For this review, take the finished solid that the model builds, in its own axes (mm). Face numbers are marked on the shaded views. A direction names the side the tool comes from. Coordinates: 2 decimals unless noted, no trailing zeros. Loops run counter-clockwise (first coordinate to the right, second up) from the corner with the lowest first, then second, coordinate; pieces in that order, holes last. Notation, with made-up numbers: (30.25, 15) - (63.25, 15) arc R37 cw to (63.25, 51) - close; hole circle Ø3 at (38.5, 46). An arc over 180 degrees is marked (long way). One line per item, written item: value. Start each with the question number.
1. The part is to be moulded in two halves that separate along Z. For the marked faces 3, 4 and 5, say which applies: released by +Z, released by -Z, zero draft, split by the parting line, or undercut.
2. Take a section at D-D, the plane x = 4.25. State the section outline as (y, z) points, and give its area (3 significant figures).
3. To check wall thickness, follow line 1 (X direction, y = 0.7, z = 5); line 2 (Z direction, x = -6.5, y = 1.35); line 3 (Z direction, x = -5, y = 2.6). State the ranges of each line that lie inside material, in increasing order. Write a range as from..to.
4. Take a section at B-B, the plane z = 5. Count the separate pieces of the cut face and the enclosed holes in it, and give its area (3 significant figures).
5. Take a section at C-C, the plane x = -1.25. State the section outline as (y, z) points, and give its area (3 significant figures).
6. Take a section at A-A, the plane y = 0.75. State the section outline as (x, z) points, and give its area (3 significant figures).
7. For the marked faces 1 and 2, list the 3-axis set-ups (+Z, -Z, +X, -X, +Y, -Y) from which the entire face can be reached by the end or side of a thin tool; tool diameter is ignored.
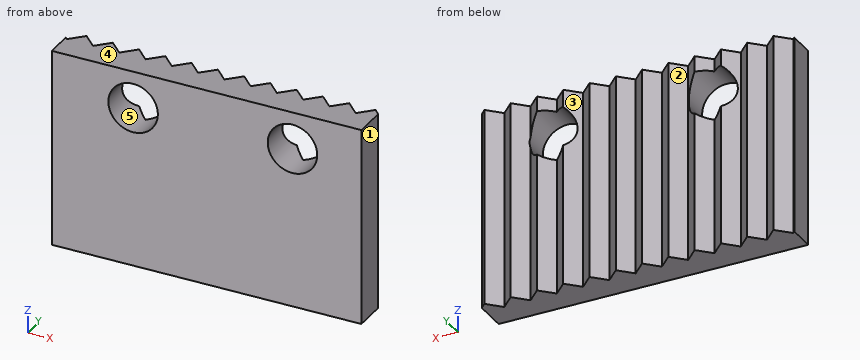
Autodesk Inventor part; units mm, degrees
ref_plane "YZ Plane" through (0, 0, 0) normal (1, 0, 0) x (0, 1, 0)
ref_plane "XZ Plane" through (0, 0, 0) normal (0, 1, 0) x (-1, 0, 0)
ref_plane "XY Plane" through (0, 0, 0) normal (0, 0, 1) x (1, 0, 0)
sketch "Sketch1" plane through (0, 0, 0) normal (0, 1, 0) x (-1, 0, 0)
  line L0 (24, 8) -> (-24, 8)
  line L1 (-24, 8) -> (-24, -8)
  line L2 (-24, -8) -> (24, -8)
  line L3 (24, -8) -> (24, 8)
  point P0 (0, 0)
  dimension "d0" = 48
  dimension "d1" = 16
extrude "Extrusion1" add sketch "Sketch1" along normal blind 2
sketch "Sketch2" plane through (-24, 0, 8) normal (0, 0, 1) x (1, 0, 0)
  line L0 (0, 2) -> (1.5, 2) construction
  line L1 (0, 3.0607) -> (1.0607, 2)
  line L2 (0, 2) -> (48, 2)
  line L3 (0, 3.0607) -> (0, 2)
  line L4 (1.0607, 2) -> (2.1213, 3.0607)
  line L5 (1.0607, 2) -> (2.5607, 2) construction
  line L6 (2.1213, 3.0607) -> (3.182, 2)
  line L7 (3.182, 2) -> (4.2426, 3.0607)
  line L8 (4.2426, 3.0607) -> (5.3033, 2)
  line L9 (5.3033, 2) -> (6.364, 3.0607)
  line L10 (6.364, 3.0607) -> (7.4246, 2)
  line L11 (7.4246, 2) -> (8.4853, 3.0607)
  line L12 (7.4246, 2) -> (8.9246, 2) construction
  line L13 (8.4853, 3.0607) -> (9.5459, 2)
  line L14 (9.5459, 2) -> (10.6066, 3.0607)
  line L15 (10.6066, 3.0607) -> (11.6673, 2)
  line L16 (11.6673, 2) -> (12.7279, 3.0607)
  line L17 (12.7279, 3.0607) -> (13.7886, 2)
  line L18 (13.7886, 2) -> (14.8492, 3.0607)
  line L19 (14.8492, 3.0607) -> (15.9099, 2)
  line L20 (15.9099, 2) -> (16.9706, 3.0607)
  line L21 (16.9706, 3.0607) -> (18.0312, 2)
  line L22 (18.0312, 2) -> (19.0919, 3.0607)
  line L23 (19.0919, 3.0607) -> (20.1525, 2)
  line L24 (20.1525, 2) -> (21.2132, 3.0607)
  line L25 (21.2132, 3.0607) -> (22.2739, 2)
  line L26 (22.2739, 2) -> (23.3345, 3.0607)
  line L27 (23.3345, 3.0607) -> (24.3952, 2)
  line L28 (24.3952, 2) -> (25.4558, 3.0607)
  line L29 (25.4558, 3.0607) -> (26.5165, 2)
  line L30 (26.5165, 2) -> (27.5772, 3.0607)
  line L31 (27.5772, 3.0607) -> (28.6378, 2)
  line L32 (27.5772, 3.0607) -> (29.0772, 3.0607) construction
  line L33 (28.6378, 2) -> (29.6985, 3.0607)
  line L34 (29.6985, 3.0607) -> (30.7591, 2)
  line L35 (30.7591, 2) -> (31.8198, 3.0607)
  line L36 (31.8198, 3.0607) -> (32.8805, 2)
  line L37 (32.8805, 2) -> (33.9411, 3.0607)
  line L38 (33.9411, 3.0607) -> (35.0018, 2)
  line L39 (35.0018, 2) -> (36.0624, 3.0607)
  line L40 (36.0624, 3.0607) -> (37.1231, 2)
  line L41 (37.1231, 2) -> (38.1838, 3.0607)
  line L42 (38.1838, 3.0607) -> (39.2444, 2)
  line L43 (39.2444, 2) -> (40.3051, 3.0607)
  line L44 (40.3051, 3.0607) -> (41.3657, 2)
  line L45 (41.3657, 2) -> (42.4264, 3.0607)
  line L46 (42.4264, 3.0607) -> (43.4871, 2)
  line L47 (43.4871, 2) -> (44.5477, 3.0607)
  line L48 (44.5477, 3.0607) -> (45.6084, 2)
  line L49 (45.6084, 2) -> (46.669, 3.0607)
  line L50 (46.669, 3.0607) -> (47.7297, 2)
  line L51 (47.7297, 2) -> (48.7904, 3.0607)
  line L52 (48, 2) -> (48, 2.2703)
  line L53 (48, 0) -> (48, 2)
  line L54 (48, 2) -> (0, 2)
  point P0 (24, 0)
  dimension "d6" = 1.5
  dimension "d7" = 1.5
  dimension "d8" = 45
  dimension "d9" = 1.5
  dimension "d10" = 1.5
  dimension "d11" = 90
  dimension "d12" = 1.5
  dimension "d13" = 1.5
  dimension "d14" = 1.5
  dimension "d15" = 1.5
  dimension "d16" = 45
  dimension "d17" = 1.5
  dimension "d18" = 90
  dimension "d19" = 1.5
  dimension "d20" = 1.5
  dimension "d21" = 1.5
  dimension "d22" = 1.5
  dimension "d23" = 1.5
  dimension "d24" = 1.5
  dimension "d25" = 90
  dimension "d26" = 1.5
  dimension "d27" = 90
  dimension "d28" = 1.5
  dimension "d29" = 90
  dimension "d30" = 1.5
  dimension "d31" = 1.5
  dimension "d32" = 1.5
  dimension "d33" = 1.5
  dimension "d34" = 90
  dimension "d35" = 1.5
  dimension "d36" = 90
  dimension "d37" = 1.5
  dimension "d38" = 90
  dimension "d39" = 1.5
  dimension "d40" = 90
  dimension "d41" = 1.5
  dimension "d42" = 90
  dimension "d43" = 1.5
  dimension "d44" = 90
  dimension "d45" = 1.5
  dimension "d46" = 45
  dimension "d47" = 1.5
  dimension "d48" = 90
  dimension "d49" = 1.5
  dimension "d50" = 90
  dimension "d51" = 1.5
  dimension "d52" = 90
  dimension "d53" = 1.5
  dimension "d54" = 90
  dimension "d55" = 1.5
  dimension "d56" = 90
  dimension "d57" = 1.5
  dimension "d58" = 90
  dimension "d59" = 1.5
  dimension "d60" = 90
  dimension "d61" = 1.5
  dimension "d62" = 90
  dimension "d63" = 1.5
  dimension "d64" = 90
  dimension "d65" = 1.5
  dimension "d66" = 90
  dimension "d67" = 1.5
  dimension "d68" = 90
  dimension "d69" = 1.5
extrude "Extrusion2" add sketch "Sketch2" against normal blind 16
sketch "Sketch4" plane through (0, 0, 0) normal (0, -1, 0) x (1, 0, 0)
  line L0 (-24, 8) -> (24, 8)
  line L1 (12.5, 8) -> (-12.5, 8)
  line L2 (-12.5, 8) -> (-12.5, -8)
  line L3 (-12.5, -8) -> (12.5, -8)
  line L4 (12.5, -8) -> (12.5, 8)
  line L5 (-12.3327, 8) -> (-12.3327, -8)
  line L6 (-12.3327, 8) -> (-24, 8)
  line L7 (-24, 8) -> (-24, -8)
  line L8 (-24, -8) -> (-12.3327, -8)
  line L9 (-12.3327, -8) -> (-12.3327, 8)
  line L10 (24, 8) -> (24, -8)
  line L11 (12.5, 8) -> (24, 8)
  line L12 (24, 8) -> (24, -8)
  line L13 (24, -8) -> (12.5, -8)
  line L14 (12.5, -8) -> (12.5, 8)
  point P0 (0, 0)
  dimension "d93" = 25
  dimension "d94" = 16
extrude "Extrusion4" cut sketch "Sketch4" against normal blind 10 contours L0 L2 L8 L7 | L0 L10 L13 L4
sketch "Sketch5" plane through (0, 0, 0) normal (0, -1, 0) x (1, 0, 0)
  circle A0 centre (6.934, 5) radius 2
  circle A1 centre (-5.934, 5) radius 2
  point P0 (0, 0)
  dimension "d97" = 4
  dimension "d98" = 4
extrude "Extrusion5" cut sketch "Sketch5" against normal blind 10
properties part number "gantryTensioner"
Solutions:
1. face 3: zero draft
1. face 4: released by +Z
1. face 5: undercut
2. outline: (0, -8) - (2.39, -8) - (2.39, 8) - (0, 8) - close
2. area: 38.2 mm2
3. line 1: -12.5..-7.93, -3.93..4.93, 8.93..12.5
3. line 2: -8..3.08, 6.92..8
3. line 3: -8..3.23, 6.77..8
4. separate pieces: 3
4. enclosed holes: 0
4. area: 42.9 mm2
5. outline: (0, -8) - (2.48, -8) - (2.48, 8) - (0, 8) - close
5. area: 39.6 mm2
6. outline: (-12.5, -8) - (12.5, -8) - (12.5, 8) - (-12.5, 8) - close; hole circle Ø4 at (-5.93, 5); hole circle Ø4 at (6.93, 5)
6. area: 375 mm2
7. face 1: +Z, -Z, +X, +Y, -Y
7. face 2: +Z, -Z, +Y
